CAD build for the part. Positions are in the model's coordinates, mm. Face numbers are marked on the shaded views. A direction names the side the tool comes from. Coordinates: 2 decimals unless noted, no trailing zeros. Write each loop counter-clockwise with the first axis right and the second up, starting at its lowest first coordinate (ties: lowest second). Pieces come first, ordered by that corner, then holes. Notation, with made-up numbers: (-35.5, -8.5) -> (-29.5, -8.5) arc R13 cw to (-29.5, 1.5) -> close; hole circle Ø9 at (76, -24). An arc over 180 degrees is marked (long way). Answer as CSV lines item,"result".
```python
from build123d import *

# Parameters (mm, degrees)
EXTRUS_O1_DEPTH = 44
CASCA1_T        = -2
EXTRUS_O2_DEPTH = 40
ESBO_O6_R       = 5.25
EXTRUS_O3_DEPTH = 2
ESBO_O5_R       = 5.25
EXTRUS_O4_DEPTH = 2
ESBO_O7_W       = 12
ESBO_O7_H       = 34
EXTRUS_O5_DEPTH = 2


with BuildPart() as part:
    # Esboço1 → Extrusão1 (new body)
    with BuildSketch(Plane(origin=(0, 0, 0), x_dir=(1, 0, 0), z_dir=(0, 1, 0))):
        Polygon((-59.5, 45.323641576), (-31, -4.676358424), (31, -4.676358424), (59.5, 45.323641576), align=None)
    extrude(amount=EXTRUS_O1_DEPTH)

    # Casca1
    casca1_openings = [part.faces().sort_by_distance(p)[0] for p in [
        (0, 22, -45.323641576),
    ]]
    offset(amount=CASCA1_T, openings=casca1_openings, kind=Kind.INTERSECTION)

    # Esboço4 → Extrusão2 (add)
    with BuildSketch(Plane.XZ.offset(-42)):
        Polygon((-57.197913989, -45.323641576), (-42.197913989, -45.323641576), (-42.197913989, -42.323641576), (-55.487913989, -42.323641576), align=None)
    extrus_o2 = extrude(amount=EXTRUS_O2_DEPTH)

    # Espelhar1: Extrusão2 across plane
    add(extrus_o2.mirror(Plane(origin=(0, 0, 0), x_dir=(0, 0, 1), z_dir=(1, 0, 0))))

    # Esboço6 → Extrusão3 (cut)
    with BuildSketch(Plane.XY.offset(-42.323641576)):
        with Locations((-49.5, 10)):
            Circle(ESBO_O6_R)
    extrus_o3 = extrude(amount=-EXTRUS_O3_DEPTH, mode=Mode.SUBTRACT)

    # Esboço5 → Extrusão4 (cut)
    with BuildSketch(Plane.XY.offset(-42.323641576)):
        with Locations((-49.5, 34)):
            Circle(ESBO_O5_R)
    extrus_o4 = extrude(amount=-EXTRUS_O4_DEPTH, mode=Mode.SUBTRACT)

    # Espelhar2: Extrusão3, Extrusão4 across plane
    add(extrus_o3.mirror(Plane(origin=(0, 0, 0), x_dir=(0, 0, 1), z_dir=(1, 0, 0))), mode=Mode.SUBTRACT)
    add(extrus_o4.mirror(Plane(origin=(0, 0, 0), x_dir=(0, 0, 1), z_dir=(1, 0, 0))), mode=Mode.SUBTRACT)

    # Esboço7 → Extrusão5 (cut)
    with BuildSketch(Plane.XY.offset(4.676358424)):
        with Locations((0, 22)):
            Rectangle(ESBO_O7_W, ESBO_O7_H)
        with Locations((19, 22)):
            Rectangle(ESBO_O7_W, ESBO_O7_H)
        with Locations((-19, 22)):
            Rectangle(ESBO_O7_W, ESBO_O7_H)
    extrude(amount=-EXTRUS_O5_DEPTH, mode=Mode.SUBTRACT)


solid = part.part
```
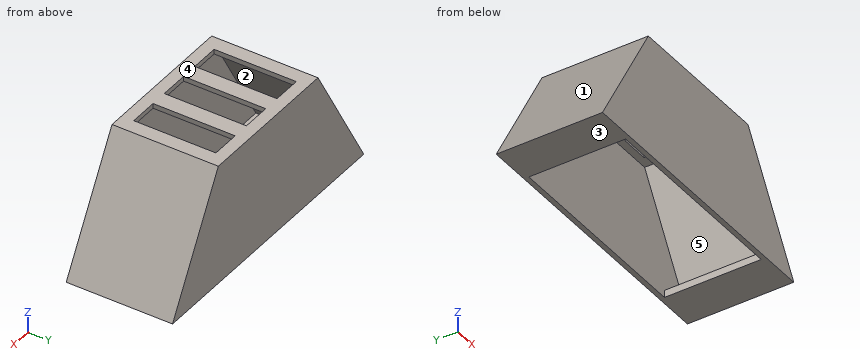
Item 1: Wall check: line 1 (Y direction, x = -49.5, z = -43.7); line 2 (Y direction, x = -33, z = -37); line 3 (Z direction, x = -9, y = 27). Give the ranges that are in metal, low to high. Write a range as from..to.
Answer below:
line 1,"y = 0..4.75, 15.25..28.75, 39.25..44"
line 2,"y = 0..2, 42..44"
line 3,"z = 2.68..4.68"
Item 2: 3-axis set-ups, long thin cutter, end or side, ignore diameter. For the marked faces 4 and 5: which of +Z, -Z, +X, -X, +Y, -Y reach the whole face in a straight line?
Answer below:
face 4,"+Z, +X, -X, +Y, -Y"
face 5,"none"
Item 3: Saw through at C-C on z = -25. Give the cut face in (x, y).
Answer below:
outline,"(-47.92, 0) -> (47.92, 0) -> (47.92, 44) -> (-47.92, 44) -> close; hole (-45.61, 2) -> (45.61, 2) -> (45.61, 42) -> (-45.61, 42) -> close"
Item 4: Saw through at D-D on x = 49.5. Give the cut face in (y, z).
Answer below:
outline,"(0, -45.32) -> (44, -45.32) -> (44, -27.78) -> (0, -27.78) -> close; hole (2, -42.32) -> (4.75, -42.32) -> (4.75, -44.32) -> (15.25, -44.32) -> (15.25, -42.32) -> (28.75, -42.32) -> (28.75, -44.32) -> (39.25, -44.32) -> (39.25, -42.32) -> (42, -42.32) -> (42, -31.82) -> (2, -31.82) -> close"
Item 5: Saw through at B-B on x = 0.5. Give the cut face in (y, z).
Answer below:
outline,"(0, -45.32) -> (2, -45.32) -> (2, 2.68) -> (5, 2.68) -> (5, 4.68) -> (0, 4.68) -> close; (39, 2.68) -> (42, 2.68) -> (42, -45.32) -> (44, -45.32) -> (44, 4.68) -> (39, 4.68) -> close"
Item 6: Two-plate mould, pull along Z, no slides. Class the marked faces 1, 2 and 3: pulls with the +Z half, pulls with the -Z half, needs draft (parallel to the pull), parting line crosses it, or undercut.
Answer below:
face 1,"pulls with the +Z half"
face 2,"undercut"
face 3,"pulls with the -Z half"
Item 7: Flat gauge pins, fed straight in: pin 1 (6.5 mm diameter, centred on x = 51, y = 13.5, fed in from +Z); pin 2 (2 mm diameter, centred on y = 7, z = -20, fed in from +X); pin 3 (5 mm diameter, centred on x = 47, y = 36, fed in from +Z). Where does each tip first touch, or does it go through?
Answer below:
pin 1,"stops at z = -24.71"
pin 2,"stops at x = 45.64"
pin 3,"stops at z = -19.01"
Item 8: Saw through at A-A on y = 10. State how many separate pieces and enclosed holes the cut face has, and give its area (3 significant figures).
Answer below:
separate pieces,"4"
enclosed holes,"0"
area,"318 mm2"
